Part model, mm, in its own coordinate system. Face numbers are marked on the shaded views. Round coordinates to 2 decimals unless told otherwise and drop trailing zeros. Write each loop counter-clockwise with the first axis right and the second up, starting at its lowest first coordinate (ties: lowest second). Pieces come first, ordered by that corner, then holes. Notation, with made-up numbers: (0.25, 2.25) -> (15.25, 2.25) arc R17 ccw to (15.25, 24.25) -> close; hole circle Ø8 at (20.25, 75.25). An arc over 180 degrees is marked (long way). Use CSV: the item, a comma, the result in double quotes. Start each with the question number.
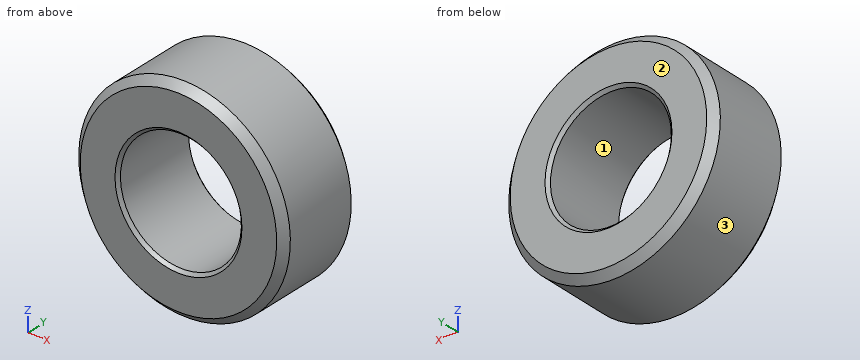
```python
from build123d import *

# Parameters (mm, degrees)
SKETCH1_R           = 7
SKETCH1_R_2         = 4
BOSS_EXTRUDE1_DEPTH = 6
CHAMFER1_SIZE       = 0.5
CHAMFER2_SIZE       = 0.2


with BuildPart() as part:
    # Sketch1 → Boss-Extrude1 (new body)
    with BuildSketch(Plane(origin=(0, 0, 0), x_dir=(1, 0, 0), z_dir=(0, 1, 0))):
        with Locations(Location((0, 0, 0), (0, 0, 270))):
            Circle(SKETCH1_R)
        with Locations(Location((0, 0, 0), (0, 0, 270))):
            Circle(SKETCH1_R_2, mode=Mode.SUBTRACT)
    extrude(amount=BOSS_EXTRUDE1_DEPTH)

    # Chamfer1
    chamfer1_edges = [part.edges().sort_by_distance(p)[0] for p in [
        (0, 0, -7),
        (0, 6, -7),
    ]]
    chamfer(chamfer1_edges, length=CHAMFER1_SIZE)

    # Chamfer2
    chamfer2_edges = [part.edges().sort_by_distance(p)[0] for p in [
        (0, 0, -4),
        (0, 6, -4),
    ]]
    chamfer(chamfer2_edges, length=CHAMFER2_SIZE)


solid = part.part
```
1. Band-saw the part on C-C (y = 1). List the corners of the cut face in (x, z), then the cut area to 3 significant figures.
2. Band-saw the part on B-B (z = 0). List the corners of the cut face in (x, y), then the cut area to 3 significant figures.
3. Pull direction X, two halves, no side cores. Call the marked faces 1, 2 and 3: released by +X, released by -X, zero draft, split by the parting line, or undercut.
4. Band-saw the part on A-A (x = 0). List the corners of the cut face in (y, z).
5. Flat gauge pins, fed straight in: pin 1 (3 mm diameter, centred on y = 1, z = 4, fed in from -X); pin 2 (1.5 mm diameter, centred on y = 5, z = 1, fed in from -X). Where does each tip first touch, or does it go through?
6. Drill centre lines: line 1 along X through (y, z) = (3.1, 0); line 2 along Z through (x, y) = (-1.25, 1.45); line 3 along Z through (x, y) = (-1, 0.6). Where is each one in solid material? Low to high. Write a range as [from, to].
Answers below:
1,outline,"circle Ø14 at (0, 0); hole circle Ø8 at (0, 0)"
1,area,"104 mm^2"
2,outline,"(-7, 0.5) -> (-6.5, 0) -> (-4.2, 0) -> (-4, 0.2) -> (-4, 5.8) -> (-4.2, 6) -> (-6.5, 6) -> (-7, 5.5) -> close; (4, 0.2) -> (4.2, 0) -> (6.5, 0) -> (7, 0.5) -> (7, 5.5) -> (6.5, 6) -> (4.2, 6) -> (4, 5.8) -> close"
2,area,"35.4 mm^2"
3,face 1,"undercut"
3,face 2,"zero draft"
3,face 3,"split by the parting line"
4,outline,"(0, -6.5) -> (0.5, -7) -> (5.5, -7) -> (6, -6.5) -> (6, -4.2) -> (5.8, -4) -> (0.2, -4) -> (0, -4.2) -> close; (0, 4.2) -> (0.2, 4) -> (5.8, 4) -> (6, 4.2) -> (6, 6.5) -> (5.5, 7) -> (0.5, 7) -> (0, 6.5) -> close"
5,pin 1,"stops at x = -6.54"
5,pin 2,"stops at x = -7"
6,line 1,"x = [-7, -4], [4, 7]"
6,line 2,"z = [-6.89, -3.8], [3.8, 6.89]"
6,line 3,"z = [-6.93, -3.87], [3.87, 6.93]"
